Can you work these out from the model? Positions are in its coordinate system, mm. A direction names the side the tool comes from. Give positions to 0.01 mm unless a question says otherwise; leave off trailing zeros. Loops run counter-clockwise (first coordinate to the right, second up) from the corner with the lowest first, then second, coordinate; pieces in that order, holes last. Notation, with made-up numbers: (61, -9) - (120, -9) arc R31 cw to (120, 25) - close; hole circle Ø3 at (44.25, 45.25). An arc over 180 degrees is marked (long way). Use a Markdown table: item, result. Add a question column.
```python
from build123d import *

# Parameters (mm, degrees)
F1_DEPTH = 20


with BuildPart() as f1:
    # F0 (on Top) → F1 (new body)
    with BuildSketch(Plane.XY):
        with BuildLine():
            Line((10, 10), (10, 0))
            Line((10, 0), (11.03011, 0))
            ThreePointArc((11.03011, 0), (14.565644, 1.464466), (16.03011, 5))
            Line((16.03011, 5), (16.03011, 18.067016))
            ThreePointArc((16.03011, 18.067016), (15.640302, 20.00251), (14.531656, 21.636215))
            ThreePointArc((14.531656, 21.636215), (0, 27.574139), (-14.531656, 21.636215))
            ThreePointArc((-14.531656, 21.636215), (-15.640302, 20.00251), (-16.03011, 18.067016))
            Line((-16.03011, 18.067016), (-16.03011, 5))
            ThreePointArc((-16.03011, 5), (-14.565644, 1.464466), (-11.03011, 0))
            Line((-11.03011, 0), (-10, 0))
            Line((-10, 0), (-10, 10))
            Line((-10, 10), (10, 10))
        make_face()
        with BuildLine():
            ThreePointArc((5.831695, 13.162136), (0, 10.311049), (-5.831695, 13.162136))
            Line((-5.831695, 13.162136), (-10, 13.162136))
            Line((-10, 13.162136), (-12.94002, 17.460051))
            ThreePointArc((-12.94002, 17.460051), (-9.572312, 20.569517), (-5.487801, 22.649662))
            ThreePointArc((-5.487801, 22.649662), (0, 25.090452), (5.487801, 22.649662))
            ThreePointArc((5.487801, 22.649662), (9.572312, 20.569517), (12.94002, 17.460051))
            Line((12.94002, 17.460051), (10, 13.162136))
            Line((10, 13.162136), (5.831695, 13.162136))
        make_face(mode=Mode.SUBTRACT)
        with BuildLine():
            ThreePointArc((2.065368, 13.162136), (0, 12.714292), (-2.065368, 13.162136))
            Line((-2.065368, 13.162136), (-5.831695, 13.162136))
            ThreePointArc((-5.831695, 13.162136), (0, 10.311049), (5.831695, 13.162136))
            Line((5.831695, 13.162136), (2.065368, 13.162136))
        make_face()
        with BuildLine():
            ThreePointArc((5.487801, 22.649662), (0, 25.090452), (-5.487801, 22.649662))
            ThreePointArc((-5.487801, 22.649662), (0, 23.574139), (5.487801, 22.649662))
        make_face()
        with BuildLine():
            ThreePointArc((-2.065368, 13.162136), (-2.698694, 21.893818), (4.986458, 17.70075))
            ThreePointArc((4.986458, 17.70075), (4.193068, 15.002057), (2.065368, 13.162136))
            Line((2.065368, 13.162136), (5.831695, 13.162136))
            ThreePointArc((5.831695, 13.162136), (6.989355, 15.301459), (7.389702, 17.70075))
            ThreePointArc((7.389702, 17.70075), (6.897858, 20.351644), (5.487801, 22.649662))
            ThreePointArc((5.487801, 22.649662), (0, 23.574139), (-5.487801, 22.649662))
            ThreePointArc((-5.487801, 22.649662), (-7.384852, 17.968429), (-5.831695, 13.162136))
            Line((-5.831695, 13.162136), (-2.065368, 13.162136))
        make_face()
    extrude(amount=F1_DEPTH)


solid = f1.part
```
1. Suppose I cut it at B-B (x = 0). List the corners of the cut face in (y, z) for me, and give its area (3 significant figures).
2. Suppose I cut it at C-C (y = 7.25). List the corners of the cut face in (x, z) for me.
3. Suppose I cut it at A-A (z = 9.5). List the corners of the cut face in (x, y) for me, and give its area (3 significant figures).
4. On a 3-axis mill with a long thin cutter (end or side, diameter ignored), from which of +Z, -Z, +X, -X, +Y, -Y can I reach the whole of each face in a straight line? I mean faces 5 (the face through (11.49, 15.34, 9.86)), 6 (the face through (10, 5, 10)), 7 (the face through (0, 11, 0)). Say none if no direction works.
5. Will these pins go through, and if not, where does the flat tip stop? P1, Ø8, axis at x = 0, y = 17.7, coming from the -Z side; P2, Ø1.3, axis at x = 7.5, z = 5, coming from the +Y side; P3, Ø4.5, axis at x = -7, z = 15, coming from the +Y side; P4, Ø2, axis at x = 0.5, z = 3, coming from the -Y side.
6. Suppose I cut it at D-D (y = 15). List the corners of the cut face in (x, z) for me, and give its area (3 significant figures).
7. If we mould it in two halves opening along X, with no side actions, what happens to faces 1 (the face through (0, 10, 10)), 2 (the face through (14.5, 1.4, 9.9)), 3 (the face through (0.225, 27.573, 9.86)), 4 (the face through (9.519, 20.606, 9.86))? For each: released by +X, released by -X, zero draft, split by the parting line, or undercut.
8. Please list where these lines run through material, in increasing order: line 1 along Y through (x, z) = (0, 10.75); line 2 along X through (y, z) = (13.5, 4); line 3 along X through (y, z) = (16, 1.75). Write a range as [from, to].
Results below:
| question | item | result |
|---|---|---|
| 1 | outline | (10, 0) - (12.71, 0) - (12.71, 20) - (10, 20) - close; (22.69, 0) - (27.57, 0) - (27.57, 20) - (22.69, 20) - close |
| 1 | area | 152 mm² |
| 2 | outline | (-16.03, 0) - (-10, 0) - (-10, 20) - (-16.03, 20) - close; (10, 0) - (16.03, 0) - (16.03, 20) - (10, 20) - close |
| 3 | outline | (-16.03, 5) arc R5 ccw to (-11.03, 0) - (-10, 0) - (-10, 10) - (10, 10) - (10, 0) - (11.03, 0) arc R5 ccw to (16.03, 5) - (16.03, 18.07) arc R5 ccw to (14.53, 21.64) arc R20.75 ccw to (-14.53, 21.64) arc R5 ccw to (-16.03, 18.07) - close; hole (-12.94, 17.46) - (-10, 13.16) - (-5.83, 13.16) arc R7.39 cw to (-5.49, 22.65) arc R16.75 ccw to start; hole (-2.07, 13.16) arc R4.99 ccw to (2.07, 13.16) arc R4.99 ccw (long way) to start; hole (5.49, 22.65) arc R7.39 cw to (7.39, 17.7) arc R7.39 cw to (5.83, 13.16) - (10, 13.16) - (12.94, 17.46) arc R16.75 ccw to start |
| 3 | area | 448 mm² |
| 4 | face 5 | +Z, -Z |
| 4 | face 6 | +Z, -Z, -Y |
| 4 | face 7 | -Z, +X, -X, +Y, -Y |
| 5 | P1 | through |
| 5 | P2 | y = 26.41 |
| 5 | P3 | y = 27.02 |
| 5 | P4 | y = 10 |
| 6 | outline | (-16.03, 0) - (-11.26, 0) - (-11.26, 20) - (-16.03, 20) - close; (-6.88, 0) - (-4.19, 0) - (-4.19, 20) - (-6.88, 20) - close; (4.19, 0) - (6.88, 0) - (6.88, 20) - (4.19, 20) - close; (11.26, 0) - (16.03, 0) - (16.03, 20) - (11.26, 20) - close |
| 6 | area | 298 mm² |
| 7 | face 1 | undercut |
| 7 | face 2 | released by +X |
| 7 | face 3 | split by the parting line |
| 7 | face 4 | undercut |
| 8 | line 1 | [10, 12.71], [22.69, 27.57] |
| 8 | line 2 | [-16.03, -10.23], [-6.08, -2.69], [2.69, 6.08], [10.23, 16.03] |
| 8 | line 3 | [-16.03, -11.94], [-7.19, -4.69], [4.69, 7.19], [11.94, 16.03] |
